Can you work these out from the model? Positions are in its coordinate system, mm. Face numbers are marked on the shaded views. A direction names the side the tool comes from. Coordinates: 2 decimals unless noted, no trailing zeros. Order: outer loops, then holes, each group sorted by start corner. A loop starts at its lowest first (then second) coordinate and runs counter-clockwise, first axis right, second up.
```python
from build123d import *
from build123d.topology import SkipClean

# Parameters (mm, degrees)
SKETCH1_W           = 54.4
SKETCH1_H           = 38.8
BOSS_EXTRUDE1_DEPTH = 3.175
SKETCH2_W           = 7
SKETCH2_H           = 15.875
BOSS_EXTRUDE2_DEPTH = 20
SKETCH3_R           = 3.8354
SKETCH3_R_2         = 2.2479
BOSS_EXTRUDE3_DEPTH = 3.175
LPATTERN1_COUNT     = 2
LPATTERN1_PITCH     = 27.94
SKETCH6_R           = 3.8354
SKETCH6_R_2         = 2.2479
BOSS_EXTRUDE6_DEPTH = 3.175
SKETCH7_R           = 2.150000018
CUT_EXTRUDE1_DEPTH  = 15.875
BOSS_EXTRUDE7_DEPTH = 1.2948
SKETCH11_R          = 2.2479
BOSS_EXTRUDE8_DEPTH = 3.175
CUT_EXTRUDE2_REACH  = 79.746
SKETCH13_W          = 3.175
SKETCH13_H          = 20
FILLET1_R           = 1.5875


with BuildPart() as part:
    # Sketch1 → Boss-Extrude1 (new body)
    with BuildSketch(Plane(origin=(0, 0, 0), x_dir=(1, 0, 0), z_dir=(0, 1, 0))):
        with Locations((27.2, 19.4)):
            Rectangle(SKETCH1_W, SKETCH1_H)
    extrude(amount=BOSS_EXTRUDE1_DEPTH)

    # Sketch2 → Boss-Extrude2 (add)
    with BuildSketch(Plane(origin=(0, 3.175, 0), x_dir=(1, 0, 0), z_dir=(0, 1, 0))):
        with Locations((3.5, 20.0625)):
            Rectangle(SKETCH2_W, SKETCH2_H)
    boss_extrude2 = extrude(amount=BOSS_EXTRUDE2_DEPTH)

    # Mirror1: Boss-Extrude2 across plane
    add(boss_extrude2.mirror(Plane.ZY.offset(-27.2)))

    # Sketch3 → Boss-Extrude3 (add)
    # profile 1 of 2: a face of its own
    with BuildSketch(Plane(origin=(0, 3.175, 0), x_dir=(1, 0, 0), z_dir=(0, 1, 0))):
        with Locations((13.109999942, -7.608)):
            Circle(SKETCH3_R)
        with Locations(Location((13.109999942, -7.608, 0), (0, 0, 270))):
            Circle(SKETCH3_R_2, mode=Mode.SUBTRACT)
    # profile 2 of 2: a face of its own
    with BuildSketch(Plane(origin=(0, 3.175, 0), x_dir=(1, 0, 0), z_dir=(0, 1, 0))):
        with BuildLine():
            Line((9.274599942, 0), (9.274599942, -7.608))
            ThreePointArc((9.274599942, -7.608), (13.109999942, -3.7726), (16.945399942, -7.608))
            Line((16.945399942, -7.608), (16.945399942, 0))
            Line((16.945399942, 0), (9.274599942, 0))
        make_face()
    boss_extrude3 = extrude(amount=-BOSS_EXTRUDE3_DEPTH)

    # LPattern1: Boss-Extrude3 ×2
    with Locations(*[(i * LPATTERN1_PITCH, 0, 0) for i in range(1, LPATTERN1_COUNT)]):
        add(boss_extrude3)

    # Sketch6 → Boss-Extrude6 (add)
    # profile 1 of 2: a face of its own
    with BuildSketch(Plane(origin=(0, 3.175, 0), x_dir=(1, 0, 0), z_dir=(0, 1, 0))):
        with Locations((4.1402, 43.7)):
            Circle(SKETCH6_R)
        with Locations(Location((4.1402, 43.7, 0), (0, 0, 270))):
            Circle(SKETCH6_R_2, mode=Mode.SUBTRACT)
    # profile 2 of 2: a face of its own
    with BuildSketch(Plane(origin=(0, 3.175, 0), x_dir=(1, 0, 0), z_dir=(0, 1, 0))):
        with BuildLine():
            ThreePointArc((7.9756, 43.7), (4.1402, 39.8646), (0.3048, 43.7))
            Line((0.3048, 43.7), (0.3048, 38.8))
            Line((0.3048, 38.8), (7.9756, 38.8))
            Line((7.9756, 38.8), (7.9756, 43.7))
        make_face()
    boss_extrude6 = extrude(amount=-BOSS_EXTRUDE6_DEPTH)

    # Mirror3: Boss-Extrude6 across plane
    add(boss_extrude6.mirror(Plane.ZY.offset(-27.2)))

    # Sketch7 → Cut-Extrude1 (cut)
    with BuildSketch(Plane(origin=(0, 0, -28), x_dir=(-1, 0, 0), z_dir=(0, 0, -1))):
        with Locations((-2.852600116, 17.925)):
            Circle(SKETCH7_R)
        with Locations((-2.852600116, 8.425)):
            Circle(SKETCH7_R)
    cut_extrude1 = extrude(amount=-CUT_EXTRUDE1_DEPTH, mode=Mode.SUBTRACT)

    # Sketch9 → Boss-Extrude7 (add)
    with BuildSketch(Plane.ZY):
        Polygon((-38.8, 0), (-38.8, 3.175), (-28, 3.175), (-28, 23.175), (-12.125, 23.175), (-12.125, 3.175), (0, 3.175), (0, 0), align=None)
    boss_extrude7 = extrude(amount=BOSS_EXTRUDE7_DEPTH)

    # Mirror4: Boss-Extrude7 across plane
    add(boss_extrude7.mirror(Plane.ZY.offset(-27.2)))

    # Mirror5: Cut-Extrude1 across plane
    add(cut_extrude1.mirror(Plane.ZY.offset(-27.2)), mode=Mode.SUBTRACT)

    # Sketch11 → Boss-Extrude8 (add)
    with SkipClean():  # the faces are left unmerged after this step: merging them gives an invalid solid
        with BuildSketch(Plane.XZ):
            with BuildLine():
                Line((0.3048, -38.8), (0.3048, -43.7))
                ThreePointArc((0.3048, -43.7), (4.1402, -47.5354), (7.9756, -43.7))
                Line((7.9756, -43.7), (7.9756, -38.8))
                Line((7.9756, -38.8), (46.4244, -38.8))
                Line((46.4244, -38.8), (46.4244, -43.7))
                ThreePointArc((46.4244, -43.7), (50.2598, -47.5354), (54.0952, -43.7))
                Line((54.0952, -43.7), (54.0952, -38.8))
                Line((54.0952, -38.8), (55.6948, -38.8))
                Line((55.6948, -38.8), (55.6948, 0))
                Line((55.6948, 0), (44.885399942, 0))
                Line((44.885399942, 0), (44.885399942, 7.608))
                ThreePointArc((44.885399942, 7.608), (41.049999942, 11.4434), (37.214599942, 7.608))
                Line((37.214599942, 7.608), (37.214599942, 0))
                Line((37.214599942, 0), (16.945399942, 0))
                Line((16.945399942, 0), (16.945399942, 7.608))
                ThreePointArc((16.945399942, 7.608), (13.109999942, 11.4434), (9.274599942, 7.608))
                Line((9.274599942, 7.608), (9.274599942, 0))
                Line((9.274599942, 0), (-1.2948, 0))
                Line((-1.2948, 0), (-1.2948, -38.8))
                Line((-1.2948, -38.8), (0.3048, -38.8))
            make_face()
            with Locations(Location((4.1402, -43.7, 0), (0, 0, 90))):
                Circle(SKETCH11_R, mode=Mode.SUBTRACT)
            with Locations(Location((50.2598, -43.7, 0), (0, 0, 90))):
                Circle(SKETCH11_R, mode=Mode.SUBTRACT)
            with Locations(Location((41.049999942, 7.608, 0), (0, 0, 90))):
                Circle(SKETCH11_R, mode=Mode.SUBTRACT)
            with Locations(Location((13.109999942, 7.608, 0), (0, 0, 90))):
                Circle(SKETCH11_R, mode=Mode.SUBTRACT)
        extrude(amount=BOSS_EXTRUDE8_DEPTH)
    add(part.part.scale(1), mode=Mode.REPLACE)  # the faces are merged on a copy

    # Sketch13 → Cut-Extrude2 (cut, up to next)
    with BuildSketch(Plane(origin=(55.6948, 0, 0), x_dir=(0, 0, -1), z_dir=(1, 0, 0)), mode=Mode.PRIVATE) as cut_extrude2_sk1:
        with Locations((13.7125, 13.175)):
            Rectangle(SKETCH13_W, SKETCH13_H)
    cut_extrude2_tool1 = extrude(cut_extrude2_sk1.sketch, amount=-CUT_EXTRUDE2_REACH, mode=Mode.PRIVATE) & part.part
    add(cut_extrude2_tool1.solids().sort_by_distance((55.6948, 13.175, -13.7125))[0], mode=Mode.SUBTRACT)

    # Fillet1
    fillet1_edges = [part.edges().sort_by_distance(p)[0] for p in [
        (-1.2948, 0, 0),
        (55.6948, 0, 0),
        (2.8526, 3.175, -12.125),
        (2.8526, 3.175, -28),
        (2.8526, 23.175, -12.125),
        (2.8526, 23.175, -28),
        (51.5474, 23.175, -15.3),
        (51.5474, 3.175, -15.3),
        (51.5474, 23.175, -28),
        (51.5474, 3.175, -28),
        (16.945399942, 0, 0),
        (9.274599942, 0, 0),
        (44.885399942, 0, 0),
        (37.214599942, 0, 0),
        (0.3048, 0, -38.8),
        (7.9756, 0, -38.8),
        (46.4244, 0, -38.8),
        (54.0952, 0, -38.8),
    ]]
    fillet(fillet1_edges, radius=FILLET1_R)


solid = part.part
```
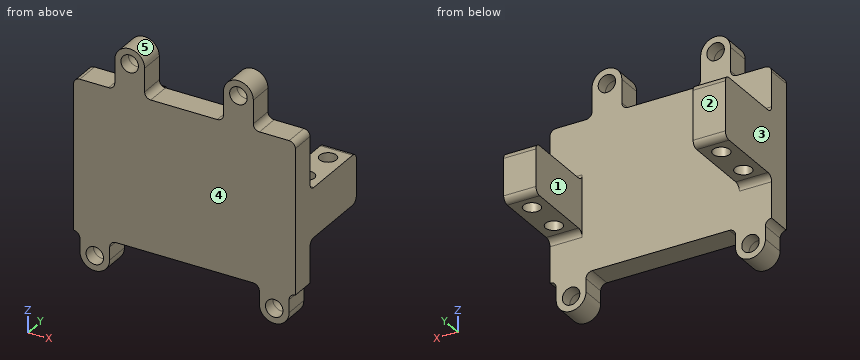
1. Thinking about a two-plate mould opening in X: for the marked faces 3, 4 and 5, which applies, pulls with the +X half, pulls with the -X half, needs draft (parallel to the pull), parting line crosses it, or undercut?
Completed:
face 3: pulls with the -X half
face 4: needs draft
face 5: undercut
2. Imagine slicing it at B-B on y = -1.5. Give the number of separate pieces and of enclosed holes in the cut face, then the cut area to 3 significant figures.
Completed:
separate pieces: 1
enclosed holes: 4
area: 2,440 mm2
3. Imagine slicing it at C-C on z = -34.5. Please give me the cut outline in (x, y) (3 decimals), then the cut area to 3 significant figures.
Completed:
outline: (-1.295, -3.175) - (55.695, -3.175) - (55.695, 3.175) - (-1.295, 3.175) - close
area: 362 mm2
4. Please list where these lines run through material, in increasing order: probe 1 along Z at (x, y) = (41.05, 1.8); probe 2 along X at (y, z) = (1, 8); probe 3 along X at (y, z) = (-2.3, -43.7).
Completed:
probe 1: z = -38.8 to 5.36, 9.86 to 11.44
probe 2: x = 9.29 to 10.9, 15.32 to 16.93, 37.23 to 38.84, 43.26 to 44.87
probe 3: x = 0.3 to 1.89, 6.39 to 7.98, 46.42 to 48.01, 52.51 to 54.1
5. I'm going to push flat-ended pins straight in: pin 1 (9 mm diameter, centred on x = 3.5, y = 15, fed in from +Z) (3 decimals); pin 2 (4 mm diameter, centred on x = 51.5, y = 9, fed in from +Z); pin 3 (1.5 mm diameter, centred on x = 37, y = 0.5, fed in from +Z); pin 4 (5 mm diameter, centred on x = 50.26, z = -43.7, fed in from -Y) (3 decimals). Where does each tip first touch, or does it pass through?
Completed:
pin 1: stops at z = -12.125
pin 2: stops at z = -15.3
pin 3: stops at z = 9.56
pin 4: stops at y = -3.175
6. Imagine slicing it at A-A on x = 41.05. Please give me the cut outline in (y, z) (3 decimals).
Completed:
outline: (-3.175, -38.8) - (3.175, -38.8) - (3.175, 5.36) - (-3.175, 5.36) - close; (-3.175, 9.856) - (3.175, 9.856) - (3.175, 11.443) - (-3.175, 11.443) - close
7. Imagine slicing it at D-D on x = 32. Please give me the cut outline in (y, z) (3 decimals).
Completed:
outline: (-3.175, -38.8) - (3.175, -38.8) - (3.175, 0) - (-3.175, 0) - close
8. On a 3-axis mill with a long thin cutter (end or side, diameter ignored), from which of +Z, -Z, +X, -X, +Y, -Y can I reach the whole of each face in a straight line? I mean the marked faces 1 and 2. Say none if no direction works.
Completed:
face 1: +Z, -Z, +Y
face 2: +Z, -Z, +X, -X, +Y
